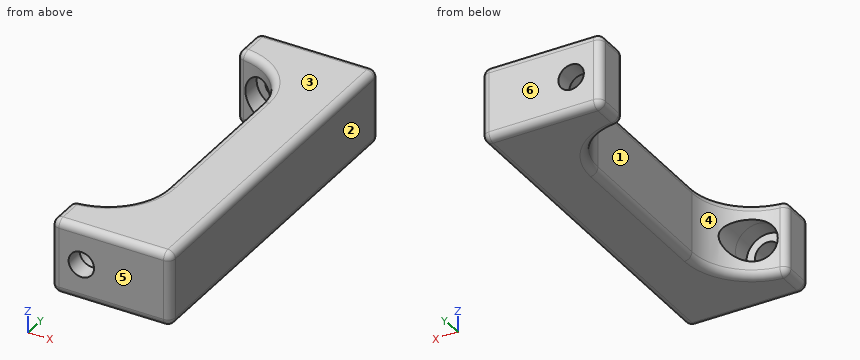
from build123d import *

# Parameters (mm, degrees)
SKETCH1_W               = 8
SKETCH1_H               = 5
SKETCH1_H_2             = 47.5
BOSS_EXTRUDE1_DEPTH     = 10
SKETCH2_R               = 1.7
CUT_EXTRUDE1_DEPTH      = 51.002499938
CUT_EXTRUDE2_DEPTH      = 40
CUT_EXTRUDE2_DEPTH_BACK = 2.5
SKETCH3_R               = 2.85
FILLET1_R               = 8
FILLET2_R               = 1


with BuildPart() as part:
    # Sketch1 → Boss-Extrude1 (new body)
    with BuildSketch(Plane.XY):
        with Locations((-8, 21.25)):
            Rectangle(SKETCH1_W, SKETCH1_H)
        Rectangle(SKETCH1_W, SKETCH1_H_2)
        with Locations((-8, -21.25)):
            Rectangle(SKETCH1_W, SKETCH1_H)
    extrude(amount=BOSS_EXTRUDE1_DEPTH)

    # Sketch2 → Cut-Extrude1 (cut, through all)
    with BuildSketch(Plane(origin=(0, 23.75, 0), x_dir=(1, 0, 0), z_dir=(0, 1, 0))):
        with Locations(Location((-8, -5, 0), (0, 0, 270))):
            Circle(SKETCH2_R)
    extrude(amount=-CUT_EXTRUDE1_DEPTH, mode=Mode.SUBTRACT)

    # Sketch3 → Cut-Extrude2 (cut, two sides: drawn at the far end of the back side and taken through both)
    with BuildSketch(Plane(origin=(0, -18.75, 0), x_dir=(1, 0, 0), z_dir=(0, 1, 0)).offset(-CUT_EXTRUDE2_DEPTH_BACK)):
        with Locations((-8, -5)):
            Circle(SKETCH3_R)
    extrude(amount=CUT_EXTRUDE2_DEPTH + CUT_EXTRUDE2_DEPTH_BACK, mode=Mode.SUBTRACT)

    # Fillet1
    # the kernel refuses this fillet: 8 mm, written as the material it adds along each edge
    with BuildSketch(Plane(origin=(-4, 18.75, 0), x_dir=(-1, 0, 0), z_dir=(0, 0, 1))) as fillet1_piece_1_section:
        with BuildLine():
            CenterArc((FILLET1_R, FILLET1_R), FILLET1_R, 180, 90)
            Line((0, FILLET1_R), (0, 0))
            Line((0, 0), (FILLET1_R, 0))
        make_face()
    fillet1_piece_1 = extrude(amount=10, mode=Mode.PRIVATE)
    fillet1_piece_1 = fillet1_piece_1 - Plane(origin=(-8, 18.525887701, 5), x_dir=(1, 0, 0), z_dir=(0, -1, 0)) * Cylinder(2.85, 53, mode=Mode.PRIVATE)
    add(fillet1_piece_1)
    with BuildSketch(Plane(origin=(-4, -18.75, 0), x_dir=(0, 1, 0), z_dir=(0, 0, 1))) as fillet1_piece_2_section:
        with BuildLine():
            CenterArc((FILLET1_R, FILLET1_R), FILLET1_R, 180, 90)
            Line((0, FILLET1_R), (0, 0))
            Line((0, 0), (FILLET1_R, 0))
        make_face()
    fillet1_piece_2 = extrude(amount=10, mode=Mode.PRIVATE)
    fillet1_piece_2 = fillet1_piece_2 - Plane(origin=(-8, -12.833542895, 5), x_dir=(1, 0, 0), z_dir=(0, 1, 0)) * Cylinder(2.85, 53, mode=Mode.PRIVATE)
    add(fillet1_piece_2)

    # Fillet2
    fillet2_edges = [part.edges().sort_by_distance(p)[0] for p in [
        (4, 0, 0),
        (-4, -23.75, 0),
        (-12, -21.25, 0),
        (-12, 21.25, 10),
        (-12, 21.25, 0),
        (-4, 23.75, 0),
        (4, 23.75, 5),
        (4, -23.75, 5),
        (-12, -23.75, 5),
        (-12, -18.75, 5),
        (-12, 18.75, 5),
        (-12, 23.75, 5),
        (-12, -21.25, 10),
        (-4, -23.75, 10),
        (4, 0, 10),
        (-4, 23.75, 10),
        (-4, 0, 0),
        (-4, 0, 10),
        (-6.343145751, 16.406854249, 0),
        (-6.343145751, 16.406854249, 10),
        (-6.343145751, -16.406854249, 0),
        (-6.343145751, -16.406854249, 10),
    ]]
    fillet(fillet2_edges, radius=FILLET2_R)


solid = part.part
Could you check a few things on this model? Use its own coordinates, in mm. Face numbers are marked on the shaded views. A direction names the side the tool comes from. Give positions to 0.01 mm unless a question says otherwise; leave off trailing zeros. Order: outer loops, then holes, each group sorted by start corner. A loop starts at its lowest first (then second) coordinate and runs counter-clockwise, first axis right, second up. Notation, with made-up numbers: (7.25, -35.75) - (50.25, -35.75) arc R18 ccw to (50.25, -4.75) - close; hole circle Ø2 at (76.5, 10.25). An arc over 180 degrees is marked (long way). One line per item, written item: value. Start each with the question number.
1. Thinking about a two-plate mould opening in Y: for the marked faces 3, 4, 5 and 6, which applies, +Y half, -Y half, draft (parallel to the pull), parting line (faces both ways), or undercut?
2. For P1, Ø3, axis at x = -7.5, z = 6.5, coming from the +Y side; P2, Ø4, axis at y = 8.5, z = 3.5, coming from the -X side, each with a flat end and sliding along its axis, tell me the tip position at first contact or that it passes through.
3. For the marked faces 1 and 2, which set-ups out of +Z, -Z, +X, -X, +Y, -Y let a thin tool reach every point of the face, with its end or its side?
4. Imagine slicing it at A-A on y = -7. List the corners of the cut face in (x, z) for me, plus the area to 3 significant figures.
5. If I drill on probe 1 along Y at (x, z) = (-10.75, 5); probe 2 along Z at (x, y) = (-8, -20.5); probe 3 along Y at (x, z) = (-10.75, 6), over which ranges is the centre line in solid material (lowest first)?
6. Imagine slicing it at B-B on z = 6.25. Give the number of separate pieces and of enclosed holes in the cut face, plus the area to 3 significant figures.
Values:
1. face 3: draft
1. face 4: undercut
1. face 5: -Y half
1. face 6: +Y half
2. P1: y = 23.75
2. P2: x = -4
3. face 1: +Z, -Z, -X
3. face 2: +Z, -Z, +X, +Y, -Y
4. outline: (-4, 1) arc R1 ccw to (-3, 0) - (3, 0) arc R1 ccw to (4, 1) - (4, 9) arc R1 ccw to (3, 10) - (-3, 10) arc R1 ccw to (-4, 9) - close
4. area: 79.1 mm²
5. probe 1: -23.75 to -21.25, 21.25 to 23.75
5. probe 2: 0 to 2.15, 7.85 to 10
5. probe 3: -23.75 to -18.65, 18.65 to 23.75
6. separate pieces: 3
6. enclosed holes: 0
6. area: 436 mm²
